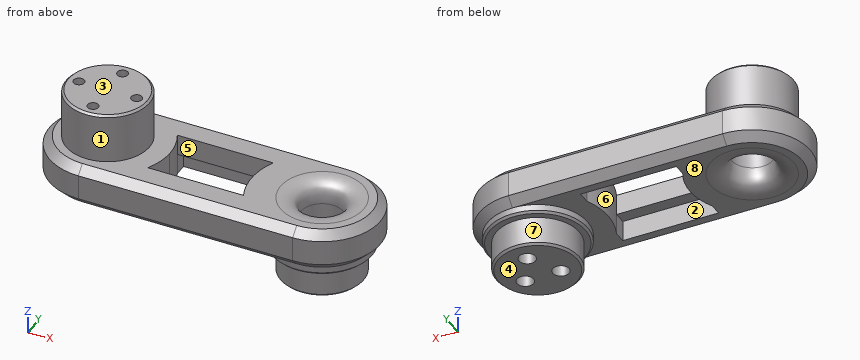
from build123d import *

# Parameters (mm, degrees)
EXTRUDE_1_DEPTH     = 10
SKETCH_2_R          = 10
EXTRUDE_2_DEPTH     = 12
SKETCH_3_R          = 10
EXTRUDE_3_DEPTH     = 9
SKETCH_4_R          = 12
SKETCH_4_R_2        = 10
EXTRUDE_4_DEPTH     = 2
CHAMFER_1_SIZE      = 0.5
CHAMFER_2_SIZE      = 2
SKETCH_5_R          = 2
CUT_EXTRUDE_1_DEPTH = 6
SKETCH_6_R          = 1.3
CUT_EXTRUDE_2_DEPTH = 6
CUT_EXTRUDE_3_DEPTH = 10
SKETCH_8_W          = 23.241567454
SKETCH_8_H          = 3
CUT_EXTRUDE_4_DEPTH = 5
SKETCH_9_R          = 5
CUT_EXTRUDE_5_DEPTH = 10
SKETCH_10_R         = 5
CUT_EXTRUDE_6_DEPTH = 10
FILLET_1_SIZE       = 5


# Some blends are built 0.0001 mm under size
with BuildPart() as part:
    # 草图1 → 凸台-拉伸1 (new body)
    with BuildSketch(Plane.XY):
        with BuildLine():
            Line((52, 14), (0, 14))
            ThreePointArc((0, 14), (-14, 0), (0, -14))
            Line((0, -14), (52, -14))
            ThreePointArc((52, -14), (66, 0), (52, 14))
        make_face()
    extrude(amount=EXTRUDE_1_DEPTH)

    # 草图2 → 凸台-拉伸2 (add)
    with BuildSketch(Plane.XY.offset(10)):
        Circle(SKETCH_2_R)
    extrude(amount=EXTRUDE_2_DEPTH)

    # 草图3 → 凸台-拉伸3 (add)
    with BuildSketch(Plane(origin=(0, 0, 0), x_dir=(-1, 0, 0), z_dir=(0, 0, -1))):
        with Locations((-52, 0)):
            Circle(SKETCH_3_R)
    extrude(amount=EXTRUDE_3_DEPTH)

    # 草图4 → 凸台-拉伸4 (add)
    with BuildSketch(Plane(origin=(0, 0, 0), x_dir=(-1, 0, 0), z_dir=(0, 0, -1))):
        with Locations(Location((-52, 0, 0), (0, 0, 180))):
            Circle(SKETCH_4_R)
        with Locations((-52, 0)):
            Circle(SKETCH_4_R_2, mode=Mode.SUBTRACT)
    extrude(amount=EXTRUDE_4_DEPTH)

    # 倒角1
    chamfer_1_edges = [part.edges().sort_by_distance(p)[0] for p in [
        (-10, 0, 22),
        (62, 0, -9),
        (40, 0, -2),
    ]]
    chamfer(chamfer_1_edges, length=CHAMFER_1_SIZE)

    # 倒角2
    chamfer_2_edges = [part.edges().sort_by_distance(p)[0] for p in [
        (66, 0, 10),
        (26, 14, 10),
        (-14, 0, 10),
        (26, -14, 10),
        (-14, 0, 0),
        (26, 14, 0),
        (66, 0, 0),
        (26, -14, 0),
    ]]
    chamfer(chamfer_2_edges, length=CHAMFER_2_SIZE - 0.0001)  # a hair under: the kernel refuses the full size

    # 草图5 → 切除-拉伸1 (cut)
    with BuildSketch(Plane(origin=(0, 0, -9), x_dir=(-1, 0, 0), z_dir=(0, 0, -1))):
        with Locations((-52, 5)):
            Circle(SKETCH_5_R)
        with Locations((-47.669872981, -2.5)):
            Circle(SKETCH_5_R)
        with Locations((-56.330127019, -2.5)):
            Circle(SKETCH_5_R)
    extrude(amount=-CUT_EXTRUDE_1_DEPTH, mode=Mode.SUBTRACT)

    # 草图6 → 切除-拉伸2 (cut)
    with BuildSketch(Plane.XY.offset(22)):
        with Locations((0, 7)):
            Circle(SKETCH_6_R)
        with Locations((7, 0)):
            Circle(SKETCH_6_R)
        with Locations((0, -7)):
            Circle(SKETCH_6_R)
        with Locations((-7, 0)):
            Circle(SKETCH_6_R)
    extrude(amount=-CUT_EXTRUDE_2_DEPTH, mode=Mode.SUBTRACT)

    # 草图7 → 切除-拉伸3 (cut)
    with BuildSketch(Plane.XY.offset(10)):
        with BuildLine():
            ThreePointArc((36.508066615, -7), (35, 0), (36.508066615, 7))
            Line((36.508066615, 7), (13.266499161, 7))
            ThreePointArc((13.266499161, 7), (14.560176637, 3.605725487), (15, 0))
            ThreePointArc((15, 0), (14.560176637, -3.605725487), (13.266499161, -7))
            Line((13.266499161, -7), (36.508066615, -7))
        make_face()
    extrude(amount=-CUT_EXTRUDE_3_DEPTH, mode=Mode.SUBTRACT)

    # 草图8 → 切除-拉伸4 (cut)
    with BuildSketch(Plane(origin=(0, 0, 0), x_dir=(-1, 0, 0), z_dir=(0, 0, -1))):
        with Locations((-24.887282888, 8.5)):
            Rectangle(SKETCH_8_W, SKETCH_8_H)
        with Locations((-24.887282888, -8.5)):
            Rectangle(SKETCH_8_W, SKETCH_8_H)
    extrude(amount=-CUT_EXTRUDE_4_DEPTH, mode=Mode.SUBTRACT)

    # 草图9 → 切除-拉伸5 (cut)
    with BuildSketch(Plane.XY.offset(10)):
        with Locations((52, 0)):
            Circle(SKETCH_9_R)
    extrude(amount=-CUT_EXTRUDE_5_DEPTH, mode=Mode.SUBTRACT)

    # 草图10 → 切除-拉伸6 (cut)
    with BuildSketch(Plane(origin=(0, 0, 0), x_dir=(-1, 0, 0), z_dir=(0, 0, -1))):
        Circle(SKETCH_10_R)
    extrude(amount=-CUT_EXTRUDE_6_DEPTH, mode=Mode.SUBTRACT)

    # 圆角1
    # a fillet whose section is not a circle: 5 mm, written as the material it takes off along each edge
    with BuildSketch(Plane(origin=(52, 0, 10), x_dir=(1, 0, 0), z_dir=(0, -1, 0))) as fillet_1_piece_1:
        with BuildLine():
            add(Edge.make_bspline([(5 + FILLET_1_SIZE, 0), (5 + FILLET_1_SIZE * 0.831801948466, 0), (5 + FILLET_1_SIZE * 0.663603896932, 0), (5 + FILLET_1_SIZE * 0.292893218813, -FILLET_1_SIZE * 0.0716919198361), (5 + FILLET_1_SIZE * 0.0716919198361, -FILLET_1_SIZE * 0.292893218813), (5, -FILLET_1_SIZE * 0.663603896932), (5, -FILLET_1_SIZE * 0.831801948466), (5, -FILLET_1_SIZE)], knots=[0, 0, 0, 0, 0, 0, 0.5, 0.5, 1, 1, 1, 1, 1, 1], degree=5))
            Line((5, -FILLET_1_SIZE), (5, 0))
            Line((5, 0), (5 + FILLET_1_SIZE, 0))
        make_face()
    revolve(axis=Axis((52, 0, 10), (0, 0, 1)), mode=Mode.SUBTRACT)
    with BuildSketch(Plane(origin=(0, 0, 0), x_dir=(-1, 0, 0), z_dir=(0, -1, 0))) as fillet_1_piece_2:
        with BuildLine():
            add(Edge.make_bspline([(5 + FILLET_1_SIZE, 0), (5 + FILLET_1_SIZE * 0.831801948466, 0), (5 + FILLET_1_SIZE * 0.663603896932, 0), (5 + FILLET_1_SIZE * 0.292893218813, -FILLET_1_SIZE * 0.0716919198361), (5 + FILLET_1_SIZE * 0.0716919198361, -FILLET_1_SIZE * 0.292893218813), (5, -FILLET_1_SIZE * 0.663603896932), (5, -FILLET_1_SIZE * 0.831801948466), (5, -FILLET_1_SIZE)], knots=[0, 0, 0, 0, 0, 0, 0.5, 0.5, 1, 1, 1, 1, 1, 1], degree=5))
            Line((5, -FILLET_1_SIZE), (5, 0))
            Line((5, 0), (5 + FILLET_1_SIZE, 0))
        make_face()
    revolve(axis=Axis((0, 0, 0), (0, 0, -1)), mode=Mode.SUBTRACT)


solid = part.part
Check sheet for the modelled part. Datum: model origin and axes. Units: mm. Face numbers are marked on the shaded views. A direction names the side the tool comes from. Give positions to 0.01 mm unless a question says otherwise; leave off trailing zeros. Order: outer loops, then holes, each group sorted by start corner. A loop starts at its lowest first (then second) coordinate and runs counter-clockwise, first axis right, second up. Notation, with made-up numbers: M 37,5.5 L 66,5.5 A26 cw 66,30.5 Z; hole C 40,45.5 d3. An arc over 180 degrees is marked long. Answer as CSV lines item,"result". Start each with the question number.
Item 1: Cross-section at D-D on z = 9. State how many separate pieces and enclosed holes the cut face has, plus the area to 3 significant figures.
Item 2: Gauge pin test, flat ends, axial feed: P1, Ø1.3, axis at x = -0.5, y = 7, coming from the +Z side; P2, Ø1, axis at x = 3, z = 0.5, coming from the -Y side; P3, Ø8, axis at y = -5.5, z = 1, coming from the +X side. Record the tip position at first contact, or that the pin passes through.
Item 3: Thickness scan on line 1 (Y direction, x = 0, z = 19.2); line 2 (X direction, y = -1.25, z = 2.5); line 3 (X direction, y = -4.25, z = 8). Record the ranges inside material, lowest first. Write a range as [from, to].
Item 4: Mould release check, pull along Y, two halves, no side actions. Record for the marked faces 6, 7 and 8: +Y half, -Y half, draft (parallel to the pull), parting line (faces both ways), or undercut.
Item 5: Tool access check on the marked faces 1, 2, 3, 4 and 5. Record the directions out of +Z, -Z, +X, -X, +Y, -Y that give a thin tool (end or side, any length) a straight path to the whole face; none if there is none.
Item 6: Cross-section at B-B on z = 18. Enter the section's corners in (x, y), plus the area to 3 significant figures.
Item 7: Cross-section at C-C on z = -7. Enter the section's corners in (x, y).
Item 8: Cross-section at A-A on x = 12. Enter the section's corners in (y, z).
Established:
1,separate pieces,"1"
1,enclosed holes,"3"
1,area,"1,390 mm^2"
2,P1,"stops at z = 16"
2,P2,"stops at y = -13"
2,P3,"stops at x = 65.91"
3,line 1,"y = [-10, -8.3], [-5.7, 5.7], [8.3, 10]"
3,line 2,"x = [-13.94, -5.13], [5.13, 14.95], [35.05, 47.16], [56.84, 65.94]"
3,line 3,"x = [-13.34, -2.63], [2.63, 14.39], [35.54, 48.55], [55.45, 65.34]"
4,face 6,"undercut"
4,face 7,"parting line"
4,face 8,"draft"
5,face 1,"+Z"
5,face 2,"-Z"
5,face 3,"+Z, +X, -X, +Y, -Y"
5,face 4,"-Z, +X, -X, +Y, -Y"
5,face 5,"+Z, -Z"
6,outline,"C 0,0 d20; hole C -7,0 d2.6; hole C 0,-7 d2.6; hole C 0,7 d2.6; hole C 7,0 d2.6"
6,area,"293 mm^2"
7,outline,"C 52,0 d20; hole C 47.67,-2.5 d4; hole C 52,5 d4; hole C 56.33,-2.5 d4"
8,outline,"M -14,2 L -12,0 L 12,0 L 14,2 L 14,8 L 12,10 L -12,10 L -14,8 Z"
